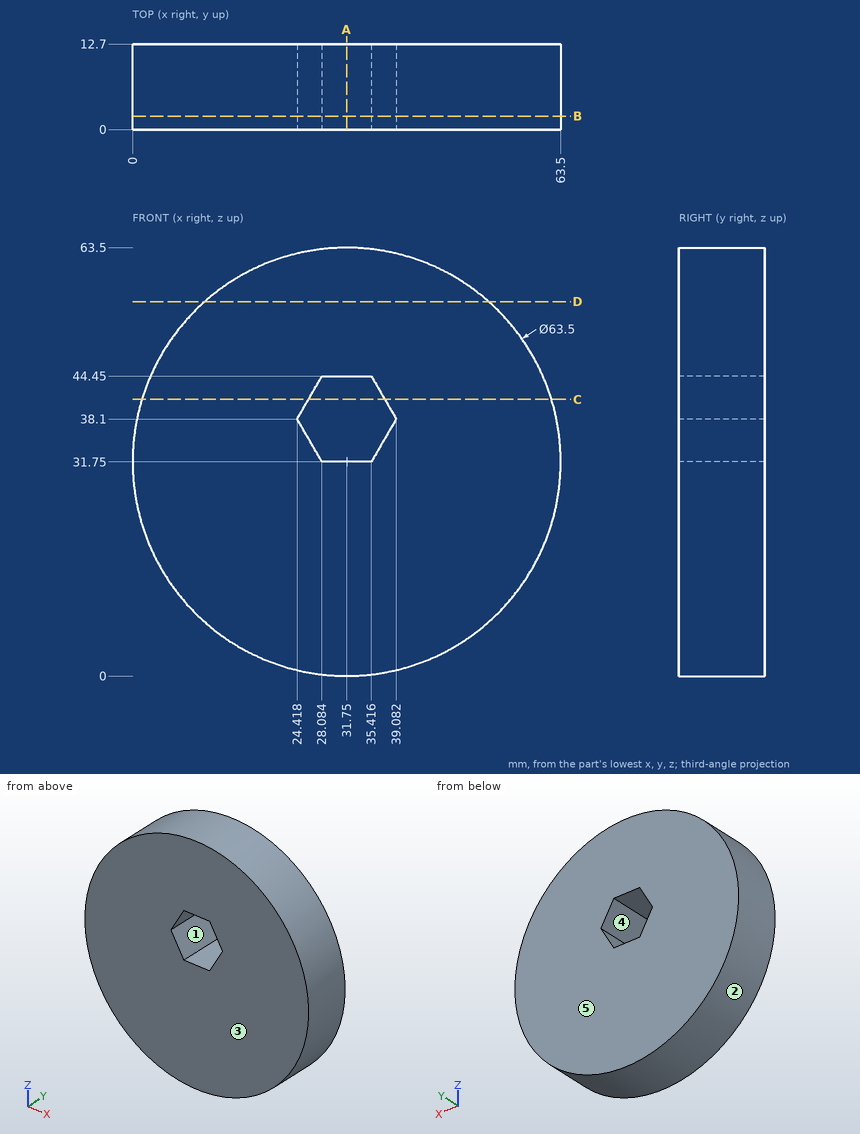
Input: dimensioned drawing with shaded views. Units: mm. Origin: part minimum x, y, z. A direction names the side the tool comes from. Round coordinates to 2 decimals unless told otherwise and drop trailing zeros. Loops run counter-clockwise (first coordinate to the right, second up) from the corner with the lowest first, then second, coordinate; pieces in that order, holes last.
1) Pin query (flat end, axial travel): pin 1 (1.5 mm diameter, centred on y = 8, z = 54, fed in from -X); pin 2 (2 mm diameter, centred on y = 1.5, z = 46, fed in from +X); pin 3 (2 mm diameter, centred on x = 39.5, z = 25, fed in from -Y); pin 4 (4 mm diameter, centred on x = 55.5, y = 2.5, fed in from -Z). Return the tip coordinate at first contact, or that it passes through.
Ans:
pin 1: stops at x = 8.39
pin 2: stops at x = 60.6
pin 3: stops at y = 0
pin 4: stops at z = 8.62
2) Section query A-A on x = 31.75. Return the cut outline in (y, z).
Ans:
outline: (0, 0) - (12.7, 0) - (12.7, 31.75) - (0, 31.75) - close; (0, 44.45) - (12.7, 44.45) - (12.7, 63.5) - (0, 63.5) - close
3) Section query D-D on z = 55.5. Return the cut outline in (x, y).
Ans:
outline: (10.68, 0) - (52.82, 0) - (52.82, 12.7) - (10.68, 12.7) - close
4) Material intervals for line 1 (Z direction, x = 32.5, y = 5.75); line 2 (Z direction, x = 30, y = 6.25); line 3 (X direction, y = 8.5, z = 31), sorted ascending.
Ans:
line 1: z = 0.01 to 31.75, 44.45 to 63.49
line 2: z = 0.05 to 31.75, 44.45 to 63.45
line 3: x = 0.01 to 63.49
5) Section query C-C on z = 41. Return the cut outline in (x, y), plus the area to 3 significant figures.
Ans:
outline: (1.38, 0) - (26.09, 0) - (26.09, 12.7) - (1.38, 12.7) - close; (37.41, 0) - (62.12, 0) - (62.12, 12.7) - (37.41, 12.7) - close
area: 628 mm2
6) Pull-direction query (X, two-part tool) for the marked faces 1, 2 and 3; classes: released by +X, released by -X, zero draft, split by the parting line, or undercut.
Ans:
face 1: undercut
face 2: split by the parting line
face 3: zero draft
7) Set-up query: the marked faces 4 and 5. Return all of +Z, -Z, +X, -X, +Y, -Y with unobstructed straight access to the full face (end or side cutting, diameter ignored); none if empty.
Ans:
face 4: +Y, -Y
face 5: +Z, -Z, +X, -X, +Y
8) Section query B-B on y = 2. Return the cut outline in (x, z), plus the area to 3 significant figures.
Ans:
outline: circle Ø63.5 at (31.75, 31.75); hole (24.42, 38.1) - (28.08, 31.75) - (35.42, 31.75) - (39.08, 38.1) - (35.42, 44.45) - (28.08, 44.45) - close
area: 3,030 mm2
